```python
from build123d import *

# Parameters (mm, degrees)
F0_W     = 137.5156
F0_H     = 68.9356
F1_DEPTH = 8.382
F2_R     = 5.08
F3_R     = 6.9215
F4_DEPTH = 1.27
F5_R     = 1.26999


# Not quite as in the source:
# - a fillet or chamfer is up to 0.001 mm smaller than in the source, because OpenCascade refuses the exact size


with BuildPart() as f1:
    # F0 (on Top) → F1 (new body)
    with BuildSketch(Plane.XY):
        Rectangle(F0_W, F0_H)
    extrude(amount=F1_DEPTH)

    # F2
    f2_edges = [f1.edges().sort_by_distance(p)[0] for p in [
        (-68.7578, 34.4678, 4.191),
        (-68.7578, -34.4678, 4.191),
        (68.7578, -34.4678, 4.191),
        (68.7578, 34.4678, 4.191),
    ]]
    fillet(f2_edges, radius=F2_R)

    # F3 (on face) → F4 (join)
    with BuildSketch(Plane(origin=(0, 0, 0), x_dir=(1, 0, 0), z_dir=(0, 0, -1))):
        with Locations((52.1843, 17.8943)):
            Circle(F3_R)
    extrude(amount=F4_DEPTH)

    # F5 (radius 1.27 in the source; OpenCascade refuses exactly that, so slightly less here)
    f5_edges = [f1.edges().sort_by_distance(p)[0] for p in [
        (45.2628, -17.8943, -1.27),
    ]]
    fillet(f5_edges, radius=F5_R)


solid = f1.part
```
Here's how the part is built. I have some questions about the finished solid (model axes, mm). Give positions to 0.01 mm unless a question says otherwise; leave off trailing zeros. Loops run counter-clockwise (first coordinate to the right, second up) from the corner with the lowest first, then second, coordinate; pieces in that order, holes last. Notation, with made-up numbers: M 42.5,37 L 92.5,37 A21 ccw 92.5,55 Z; hole C 26,54.5 d11. An arc over 180 degrees is marked long. Use one line per item in the form item = value. Start each with the question number.
Q1. I need wall thicknesses on line 1 along Z through (x, y) = (-54.5, -25.5); line 2 along Y through (x, z) = (48.5, -0.25); line 3 along X through (y, z) = (-31, 6.25). Which ranges of each line are inside material? Lowest first, please.
Q2. If we section it at B-B (x = -34.5): Write out the boundary of the cut face in (y, z), then the cut area to 3 significant figures.
Q3. If we section it at A-A (y = -5): Write out the boundary of the cut face in (x, z).
Q4. Will this pin go through, and if not, where does the flat tip stop? pin 1 Ø1 at (x, y) = (-50, -19) entering from -Z.
Taken from the geometry:
q1.line_1 = 0 to 8.38
q1.line_2 = -23.72 to -12.06
q1.line_3 = -68.5 to 68.5
q2.outline = M -34.47,0 L 34.47,0 L 34.47,8.38 L -34.47,8.38 Z
q2.area = 578 mm^2
q3.outline = M -68.76,0 L 68.76,0 L 68.76,8.38 L -68.76,8.38 Z
q4.pin_1 = 0
